from build123d import *

# Parameters (mm, degrees)
F0_R     = 508
F1_DEPTH = 38.1
F4_D     = 889
F6_DEPTH = 38.1
F7_R     = 449.2110909422
F7_R_2   = 448.3937142921
F8_DEPTH = 5.08


with BuildPart() as f1:
    # F0 (on Right) → F1 (new body)
    with BuildSketch(Plane.YZ):
        Circle(F0_R)
    extrude(amount=F1_DEPTH)

    # F4 (through all)
    with Locations(Plane.YZ.offset(38.1)):
        with Locations((0, 0)):
            Hole(F4_D / 2)

    # F5 (on face) → F6 (join)
    with BuildSketch(Plane(origin=(0, 0, 0), x_dir=(0, -1, 0), z_dir=(-1, 0, 0))):
        with BuildLine():
            ThreePointArc((444.5, 0), (333.1536714942, 294.2598871235), (54.8987348933, 441.0967908601))
            ThreePointArc((54.8987348933, 441.0967908601), (21.5516885972, 0.4157843691), (71.8712062792, -438.6510910826))
            ThreePointArc((71.8712062792, -438.6510910826), (338.767620347, -287.7789940292), (444.5, 0))
        make_face()
        with BuildLine():
            ThreePointArc((-51.3196943653, -441.5275064707), (-14.4431317717, -0.1011743755), (-57.5001694311, 440.7652215357))
            ThreePointArc((-57.5001694311, 440.7652215357), (-444.4890945371, -3.1136534152), (-51.3196943653, -441.5275064707))
        make_face()
    extrude(amount=-F6_DEPTH)

    # F7 (on face) → F8 (join)
    with BuildSketch(Plane(origin=(0, 0, 0), x_dir=(0, -1, 0), z_dir=(-1, 0, 0))):
        Circle(F7_R)
        Circle(F7_R_2, mode=Mode.SUBTRACT)
    extrude(amount=F8_DEPTH)


solid = f1.part
Verification items for the finished model (mm, model axes). A direction names the side the tool comes from. Round coordinates to 2 decimals unless told otherwise and drop trailing zeros. Loops run counter-clockwise (first coordinate to the right, second up) from the corner with the lowest first, then second, coordinate; pieces in that order, holes last. Notation, with made-up numbers: (2.5, 2.5) - (19.5, 2.5) arc R17 ccw to (19.5, 7.5) - close; hole circle Ø1 at (32, -25.5). An arc over 180 degrees is marked (long way). Answer in a Markdown table with one row per item. Add a question column.
Q1. Section check C-C on x = 28. Enter the section's corners in (y, z), plus the area to 3 significant figures.
Q2. Section check A-A on y = 0. Enter the section's corners in (x, z), plus the area to 3 significant figures.
Q3. Gauge pin test, flat ends, axial feed: pin 1 (12 mm diameter, centred on x = 8.5, z = -267, fed in from -Y); pin 2 (8 mm diameter, centred on x = 5, z = -193, fed in from -Y); pin 3 (10 mm diameter, centred on x = 22.5, z = -363, fed in from -Y). Record the tip position at first contact, or that the pin passes through.
Q4. Section check D-D on y = -102. Enter the section's corners in (x, z), plus the area to 3 significant figures.
Q5. Material ranges on line 1 (Z direction, x = -3.55, y = 0); line 2 (X direction, y = -403, z = -87); line 3 (Y direction, x = 33, z = 71), recorded low to high.
Q6. Release check for a two-part mould opening along Z. For faces 4 (the face through (18.78, -110.12, -495.92)), 5 (the face through (18.783, 14.407, -6.311)), 6 (the face through (0, -35, -449)) record: pulls with the +Z half, pulls with the -Z half, needs draft (parallel to the pull), parting line crosses it, or undercut.
Q7. Tool access check on faces 1 (the face through (18.78, -21.44, 6.61)), 2 (the face through (38.1, -106, 7)), 3 (the face through (-2.504, 356.479, -273.338)). Record the directions out of +Z, -Z, +X, -X, +Y, -Y that give a thin tool (end or side, any length) a straight path to the whole face; none if there is none.
Q8. Section check B-B on z = 82.5. Enter the section's corners in (x, y).
Found:
| question | item | result |
|---|---|---|
| 1 | outline | circle Ø1016 at (0, 0); hole (-71.87, -438.65) arc R444.5 ccw to (51.32, -441.53) arc R2454.69 cw to (57.5, 440.77) arc R444.5 ccw to (-54.9, 441.1) arc R2333.97 cw to start |
| 1 | area | 754,000 mm² |
| 2 | outline | (-5.08, -449.21) - (0, -449.21) - (0, -508) - (38.1, -508) - (38.1, -444.5) - (0, -444.5) - (0, -448.39) - (-5.08, -448.39) - close; (-5.08, 448.39) - (0, 448.39) - (0, 444.5) - (38.1, 444.5) - (38.1, 508) - (0, 508) - (0, 449.21) - (-5.08, 449.21) - close |
| 2 | area | 4,850 mm² |
| 3 | pin 1 | stops at y = -435.82 |
| 3 | pin 2 | stops at y = -471.53 |
| 3 | pin 3 | stops at y = -360.42 |
| 4 | outline | (-5.08, -437.48) - (0, -437.48) - (0, -497.65) - (38.1, -497.65) - (38.1, 497.65) - (0, 497.65) - (0, 437.48) - (-5.08, 437.48) - (-5.08, 436.64) - (0, 436.64) - (0, -436.64) - (-5.08, -436.64) - close |
| 4 | area | 37,900 mm² |
| 5 | line 1 | z = -449.21 to -448.39, 448.39 to 449.21 |
| 5 | line 2 | x = 0 to 38.1 |
| 5 | line 3 | y = -503.01 to -21.26, 15.97 to 503.01 |
| 6 | face 4 | parting line crosses it |
| 6 | face 5 | undercut |
| 6 | face 6 | needs draft |
| 7 | face 1 | +X, -X |
| 7 | face 2 | +Z, -Z, +X, +Y, -Y |
| 7 | face 3 | -X |
| 8 | outline | (-5.08, -441.57) - (0, -441.57) - (0, -501.26) - (38.1, -501.26) - (38.1, -21.41) - (0, -21.41) - (0, -440.74) - (-5.08, -440.74) - close; (-5.08, 440.74) - (0, 440.74) - (0, 16.41) - (38.1, 16.41) - (38.1, 501.26) - (0, 501.26) - (0, 441.57) - (-5.08, 441.57) - close |
